Part model, mm, in its own coordinate system. A direction names the side the tool comes from. Round coordinates to 2 decimals unless told otherwise and drop trailing zeros. Loops run counter-clockwise (first coordinate to the right, second up) from the corner with the lowest first, then second, coordinate; pieces in that order, holes last. Notation, with made-up numbers: (83, -10) -> (138, -10) arc R16 cw to (138, 14) -> close; hole circle Ø4 at (31.5, 51). An arc over 180 degrees is marked (long way). Answer as CSV lines item,"result".
from build123d import *

# Parameters (mm, degrees)
F1_DEPTH = 17
F2_T     = -1
F3_R     = 14.3708631793
F4_DEPTH = 25
F5_R     = 10.5711008848
F5_R_2   = 10.0457234784
F5_R_3   = 11.8075026786
F6_DEPTH = 17


with BuildPart() as f1:
    # F0 (on Top) → F1 (new body)
    with BuildSketch(Plane.XY):
        Polygon((-37.4681577086, -50.3954030573), (-2.5307838805, -48.2072606683), (-2.4370756, -77.2388204932), (3.3520292491, -77.2388204932), (3.3520292491, -49.0849018097), (33.674325794, -49.0849018097), (28.1071402133, -33.0383218825), (66.2586987019, -9.6234139055), (56.2705285847, -3.4012699034), (61.6739653051, 15.4289007187), (42.8437963128, 12.8090493381), (37.5377945602, 26.0640811175), (22.0817681402, 7.6640532352), (27.0145568802, 46.333488356), (13.1010971963, 39.7568419576), (0, 67.4733370543), (-13.7401381508, 40.9238524735), (-26.589423418, 48.39893803), (-20.3813649714, 4.3794875965), (-40.5914485455, 25.1100063324), (-45.4480871558, 13.568257913), (-61.4539161325, 14.2708420753), (-56.5707497299, -4.8887040466), (-63.317425549, -10.6540471315), (-31.4872264862, -36.6830341518), align=None)
    extrude(amount=F1_DEPTH)

    # F2
    f2_openings = [f1.faces().sort_by_distance(p)[0] for p in [
        (-0.409278, -4.179109, 0),
    ]]
    offset(amount=F2_T, openings=f2_openings, kind=Kind.INTERSECTION)

    # F3 (on face) → F4 (cut)
    with BuildSketch(Plane.XY.offset(17)):
        with Locations((0, -27.5635700673)):
            Circle(F3_R)
    extrude(amount=F4_DEPTH, mode=Mode.SUBTRACT)

    # F5 (on Top) → F6 (cut)
    with BuildSketch(Plane.XY):
        with Locations((0, 31.2744565308)):
            Circle(F5_R)
        with Locations((-34.3855284154, -7.6958090067)):
            Circle(F5_R_2)
        with Locations((33.7305627763, -3.4385530744)):
            Circle(F5_R_3)
    extrude(amount=F6_DEPTH, mode=Mode.SUBTRACT)


solid = f1.part
Q1. Which spindle directions (+Z, -Z, +X, -X, +Y, -Y) get a long thin tool onto all of the face, cutting with end or side? Do faces 4 (the face through (-59.897, -7.731, 8.381)), 5 (the face through (61.335, -6.556, 8.381)), 6 (the face through (2.352, -62, 8)). Say none if no direction does.
Geometry results:
face 4,"+Z, -Z, -X"
face 5,"+Z, -Z, +X"
face 6,"-Z"
Q2. Saw through at A-A, the plane y = 57.5. Write the cut outline in (x, z).
Geometry results:
outline,"(-5.16, 0) -> (-4.04, 0) -> (-4.04, 16) -> (3.61, 16) -> (3.61, 0) -> (4.71, 0) -> (4.71, 17) -> (-5.16, 17) -> close"
Q3. Saw through at B-B, the plane y = -23.5. Write the cut outline in (x, z).
Geometry results:
outline,"(-47.61, 0) -> (-46.03, 0) -> (-46.03, 16) -> (41.74, 16) -> (41.74, 0) -> (43.65, 0) -> (43.65, 17) -> (-47.61, 17) -> close"
Q4. Drill centre lines: line 1 along Y through (x, z) = (0, 16.25); line 2 along X through (y, z) = (16.5, 7); line 3 along X through (y, z) = (-71, 14.75). Where is each one in solid material? Low to high.
Geometry results:
line 1,"-77.24 to 20.7, 41.85 to 67.47"
line 2,"-44.21 to -43.13, -33.59 to -32.2, -22.09 to -21.08, 22.2 to 23.21, 29.5 to 30.81, 40.29 to 41.37"
line 3,"-2.46 to -1.46, 2.35 to 3.35"
Q5. Drop flat-ended pins along their axis: P1, Ø6, axis at x = 35, z = 13, coming from the -Y side; P2, Ø6, axis at x = 49, z = 4, coming from the +Y side; P3, Ø8, axis at y = -60.5, z = 12, coming from the -X side. Give the stop position or say it passes through.
Geometry results:
P1,"y = -49.08"
P2,"y = 14.08"
P3,"x = -2.5"
Q6. Two-plate mould, pull along Y, no slides. Class faces 1 (the face through (23.19, 24.25, 7.89)), 2 (the face through (-23, 6, 0)), 3 (the face through (18, -49.085, 8)): pulls with the +Y half, pulls with the -Y half, needs draft (parallel to the pull), parting line crosses it, or undercut.
Geometry results:
face 1,"undercut"
face 2,"needs draft"
face 3,"pulls with the -Y half"
